Read the model definition and answer for the solid it produces. Units are mm, in the model's axes. Face numbers are marked on the shaded views. A direction names the side the tool comes from. Coordinates: 2 decimals unless noted, no trailing zeros. Write each loop counter-clockwise with the first axis right and the second up, starting at its lowest first coordinate (ties: lowest second). Pieces come first, ordered by that corner, then holes. Notation, with made-up numbers: (-37, -9.75) -> (-4, -9.75) arc R28 cw to (-4, 11.25) -> close; hole circle Ø9 at (22, -38.75). An arc over 180 degrees is marked (long way). One line per item, written item: value. Start each with the question number.
1. For the marked faces 4, 5 and 6, determine the directions among +Z, -Z, +X, -X, +Y, -Y from which every point of the face is accessible in a straight line to the end or side of a thin tool.
2. Find section C-C, the plane z = 4.25. Write down the section's boundary in (x, y).
3. Given P1, Ø1, axis at x = -5.5, z = 4.5, coming from the +Y side; P2, Ø2, axis at y = 6.5, z = 3, coming from the +X side, each flat-ended and moving along its own axis, determine where each tip first touches the part or whether it passes through.
4. Consider line 1 along Y through (x, z) = (5.25, 3.25); line 2 along Y through (x, z) = (-5, 0.5); line 3 along Z through (x, y) = (-0.75, -1.75). Determine where each line is inside the solid, lowest interval first.
5. For a pull along Y with two mould halves and no side action, classify the marked faces 1, 2 and 3 as pulls with the +Y half, pulls with the -Y half, needs draft (parallel to the pull), parting line crosses it, or undercut.
6. Find section B-B, the plane x = -1. Write down the section's boundary in (y, z).
7. Find section D-D, the plane y = 7. Write down the section's boundary in (x, z), and give its area (3 significant figures).
8. Find section A-A, the plane z = 5.3. Write down the section's boundary in (x, y), and give its area (3 significant figures).
```python
from build123d import *

# Parameters (mm, degrees)
F1_DEPTH      = 3
F2_DEPTH      = 6
F4_DEPTH      = 1.5
F4_DEPTH_BACK = 1.5


with BuildPart() as f1:
    # F0 (on Top) → F1 (new body)
    with BuildSketch(Plane.XY):
        with BuildLine():
            ThreePointArc((5.811145618, 2), (5.4091097712, 4.5797958998), (7.6000000059, 6))
            Line((7.6000000059, 6), (-7.5999999941, 6))
            ThreePointArc((-7.5999999941, 6), (-5.9029437231, 5.2970562728), (-5.2, 3.6))
            ThreePointArc((-5.2, 3.6), (-5.3579863385, 2.7436269845), (-5.811145618, 2))
            Line((-5.811145618, 2), (5.811145618, 2))
        make_face()
        with BuildLine():
            ThreePointArc((7.6, -6), (8.9856406461, -5.5595917942), (9.8627416998, -4.4))
            ThreePointArc((9.8627416998, -4.4), (8.9856406461, -3.2404082058), (7.6, -2.8))
            ThreePointArc((7.6, -2.8), (6.2143593539, -3.2404082058), (5.3372583002, -4.4))
            ThreePointArc((5.3372583002, -4.4), (6.2143593539, -5.5595917942), (7.6, -6))
        make_face()
        with BuildLine():
            ThreePointArc((9.8627416998, -4.4), (9.9654365432, -4.0058447489), (10, -3.6))
            ThreePointArc((10, -3.6), (8.0058447489, -1.2345634568), (5.3372583002, -2.8))
            Line((5.3372583002, -2.8), (7.6, -2.8))
            ThreePointArc((7.6, -2.8), (8.9856406461, -3.2404082058), (9.8627416998, -4.4))
        make_face()
        with BuildLine():
            ThreePointArc((7.6, -6), (6.2143593539, -5.5595917942), (5.3372583002, -4.4))
            ThreePointArc((5.3372583002, -4.4), (5.2, -5.2), (5.3372583002, -6))
            Line((5.3372583002, -6), (7.6, -6))
        make_face()
        with BuildLine():
            ThreePointArc((-5.3372583002, -4.4), (-6.2143593453, -5.5595917881), (-7.5999999788, -6))
            Line((-7.5999999788, -6), (-5.3372583002, -6))
            ThreePointArc((-5.3372583002, -6), (-5.2345634568, -5.6058447489), (-5.2, -5.2))
            ThreePointArc((-5.2, -5.2), (-5.2345634568, -4.7941552511), (-5.3372583002, -4.4))
        make_face()
        with BuildLine():
            ThreePointArc((-7.6, -2.8), (-8.9856406461, -3.2404082058), (-9.8627416998, -4.4))
            ThreePointArc((-9.8627416998, -4.4), (-8.9856406374, -5.5595918003), (-7.5999999788, -6))
            ThreePointArc((-7.5999999788, -6), (-6.2143593453, -5.5595917881), (-5.3372583002, -4.4))
            ThreePointArc((-5.3372583002, -4.4), (-6.2143593539, -3.2404082058), (-7.6, -2.8))
        make_face()
        with BuildLine():
            ThreePointArc((-5.3372583002, -2.8), (-8.0058447489, -1.2345634568), (-10, -3.6))
            ThreePointArc((-10, -3.6), (-9.9654365432, -4.0058447489), (-9.8627416998, -4.4))
            ThreePointArc((-9.8627416998, -4.4), (-8.9856406461, -3.2404082058), (-7.6, -2.8))
            Line((-7.6, -2.8), (-5.3372583002, -2.8))
        make_face()
        with BuildLine():
            ThreePointArc((-5.2, 3.6), (-5.9029437231, 5.2970562728), (-7.5999999941, 6))
            ThreePointArc((-7.5999999941, 6), (-9.2970562728, 5.2970562769), (-10, 3.6))
            ThreePointArc((-10, 3.6), (-9.8420136615, 2.7436269845), (-9.388854382, 2))
            Line((-9.388854382, 2), (-5.811145618, 2))
            ThreePointArc((-5.811145618, 2), (-5.3579863385, 2.7436269845), (-5.2, 3.6))
        make_face()
        with BuildLine():
            ThreePointArc((10, 3.6), (9.2970562769, 5.2970562728), (7.6000000059, 6))
            ThreePointArc((7.6000000059, 6), (5.4091097712, 4.5797958998), (5.811145618, 2))
            Line((5.811145618, 2), (9.388854382, 2))
            ThreePointArc((9.388854382, 2), (9.8420136615, 2.7436269845), (10, 3.6))
        make_face()
        with BuildLine():
            ThreePointArc((5.3372583002, -4.4), (5.2, -3.6), (5.3372583002, -2.8))
            Line((5.3372583002, -2.8), (-5.3372583002, -2.8))
            ThreePointArc((-5.3372583002, -2.8), (-5.2345634568, -3.1941552511), (-5.2, -3.6))
            ThreePointArc((-5.2, -3.6), (-5.2345634568, -4.0058447489), (-5.3372583002, -4.4))
            ThreePointArc((-5.3372583002, -4.4), (-5.2345634568, -4.7941552511), (-5.2, -5.2))
            ThreePointArc((-5.2, -5.2), (-5.2345634568, -5.6058447489), (-5.3372583002, -6))
            Line((-5.3372583002, -6), (5.3372583002, -6))
            ThreePointArc((5.3372583002, -6), (5.2, -5.2), (5.3372583002, -4.4))
        make_face()
        with BuildLine():
            ThreePointArc((-5.2, -3.6), (-5.2345634568, -3.1941552511), (-5.3372583002, -2.8))
            Line((-5.3372583002, -2.8), (-7.6, -2.8))
            ThreePointArc((-7.6, -2.8), (-6.2143593539, -3.2404082058), (-5.3372583002, -4.4))
            ThreePointArc((-5.3372583002, -4.4), (-5.2345634568, -4.0058447489), (-5.2, -3.6))
        make_face()
        with BuildLine():
            Line((7.6, -2.8), (5.3372583002, -2.8))
            ThreePointArc((5.3372583002, -2.8), (5.2, -3.6), (5.3372583002, -4.4))
            ThreePointArc((5.3372583002, -4.4), (6.2143593539, -3.2404082058), (7.6, -2.8))
        make_face()
        with BuildLine():
            ThreePointArc((9.388854382, 2), (7.6, 1.2), (5.811145618, 2))
            Line((5.811145618, 2), (-5.811145618, 2))
            ThreePointArc((-5.811145618, 2), (-7.6, 1.2), (-9.388854382, 2))
            Line((-9.388854382, 2), (-10, 2))
            Line((-10, 2), (-10, -3.6))
            ThreePointArc((-10, -3.6), (-8.0058447489, -1.2345634568), (-5.3372583002, -2.8))
            Line((-5.3372583002, -2.8), (5.3372583002, -2.8))
            ThreePointArc((5.3372583002, -2.8), (8.0058447489, -1.2345634568), (10, -3.6))
            Line((10, -3.6), (10, 2))
            Line((10, 2), (9.388854382, 2))
        make_face()
        with BuildLine():
            Line((9.388854382, 2), (5.811145618, 2))
            ThreePointArc((5.811145618, 2), (7.6, 1.2), (9.388854382, 2))
        make_face()
        with BuildLine():
            ThreePointArc((-9.388854382, 2), (-7.6, 1.2), (-5.811145618, 2))
            Line((-5.811145618, 2), (-9.388854382, 2))
        make_face()
        with BuildLine():
            ThreePointArc((-9.388854382, 2), (-9.8420136615, 2.7436269845), (-10, 3.6))
            Line((-10, 3.6), (-10, 2))
            Line((-10, 2), (-9.388854382, 2))
        make_face()
        with BuildLine():
            Line((10, 2), (10, 3.6))
            ThreePointArc((10, 3.6), (9.8420136615, 2.7436269845), (9.388854382, 2))
            Line((9.388854382, 2), (10, 2))
        make_face()
    extrude(amount=F1_DEPTH)

    # F0 (on Top) → F2 (join)
    with BuildSketch(Plane.XY):
        with BuildLine():
            ThreePointArc((5.3372583002, -4.4), (5.2, -3.6), (5.3372583002, -2.8))
            Line((5.3372583002, -2.8), (-5.3372583002, -2.8))
            ThreePointArc((-5.3372583002, -2.8), (-5.2345634568, -3.1941552511), (-5.2, -3.6))
            ThreePointArc((-5.2, -3.6), (-5.2345634568, -4.0058447489), (-5.3372583002, -4.4))
            ThreePointArc((-5.3372583002, -4.4), (-5.2345634568, -4.7941552511), (-5.2, -5.2))
            ThreePointArc((-5.2, -5.2), (-5.2345634568, -5.6058447489), (-5.3372583002, -6))
            Line((-5.3372583002, -6), (5.3372583002, -6))
            ThreePointArc((5.3372583002, -6), (5.2, -5.2), (5.3372583002, -4.4))
        make_face()
        with BuildLine():
            ThreePointArc((-7.6, -2.8), (-8.9856406461, -3.2404082058), (-9.8627416998, -4.4))
            ThreePointArc((-9.8627416998, -4.4), (-8.9856406374, -5.5595918003), (-7.5999999788, -6))
            ThreePointArc((-7.5999999788, -6), (-6.2143593453, -5.5595917881), (-5.3372583002, -4.4))
            ThreePointArc((-5.3372583002, -4.4), (-6.2143593539, -3.2404082058), (-7.6, -2.8))
        make_face()
        with BuildLine():
            ThreePointArc((-5.3372583002, -4.4), (-6.2143593453, -5.5595917881), (-7.5999999788, -6))
            Line((-7.5999999788, -6), (-5.3372583002, -6))
            ThreePointArc((-5.3372583002, -6), (-5.2345634568, -5.6058447489), (-5.2, -5.2))
            ThreePointArc((-5.2, -5.2), (-5.2345634568, -4.7941552511), (-5.3372583002, -4.4))
        make_face()
        with BuildLine():
            ThreePointArc((-5.2, -3.6), (-5.2345634568, -3.1941552511), (-5.3372583002, -2.8))
            Line((-5.3372583002, -2.8), (-7.6, -2.8))
            ThreePointArc((-7.6, -2.8), (-6.2143593539, -3.2404082058), (-5.3372583002, -4.4))
            ThreePointArc((-5.3372583002, -4.4), (-5.2345634568, -4.0058447489), (-5.2, -3.6))
        make_face()
        with BuildLine():
            ThreePointArc((7.6, -6), (8.9856406461, -5.5595917942), (9.8627416998, -4.4))
            ThreePointArc((9.8627416998, -4.4), (8.9856406461, -3.2404082058), (7.6, -2.8))
            ThreePointArc((7.6, -2.8), (6.2143593539, -3.2404082058), (5.3372583002, -4.4))
            ThreePointArc((5.3372583002, -4.4), (6.2143593539, -5.5595917942), (7.6, -6))
        make_face()
        with BuildLine():
            ThreePointArc((7.6, -6), (6.2143593539, -5.5595917942), (5.3372583002, -4.4))
            ThreePointArc((5.3372583002, -4.4), (5.2, -5.2), (5.3372583002, -6))
            Line((5.3372583002, -6), (7.6, -6))
        make_face()
        with BuildLine():
            Line((7.6, -2.8), (5.3372583002, -2.8))
            ThreePointArc((5.3372583002, -2.8), (5.2, -3.6), (5.3372583002, -4.4))
            ThreePointArc((5.3372583002, -4.4), (6.2143593539, -3.2404082058), (7.6, -2.8))
        make_face()
        with BuildLine():
            ThreePointArc((-5.2, 3.6), (-5.9029437231, 5.2970562728), (-7.5999999941, 6))
            ThreePointArc((-7.5999999941, 6), (-9.2970562728, 5.2970562769), (-10, 3.6))
            ThreePointArc((-10, 3.6), (-9.8420136615, 2.7436269845), (-9.388854382, 2))
            Line((-9.388854382, 2), (-5.811145618, 2))
            ThreePointArc((-5.811145618, 2), (-5.3579863385, 2.7436269845), (-5.2, 3.6))
        make_face()
        with BuildLine():
            ThreePointArc((5.811145618, 2), (5.4091097712, 4.5797958998), (7.6000000059, 6))
            Line((7.6000000059, 6), (-7.5999999941, 6))
            ThreePointArc((-7.5999999941, 6), (-5.9029437231, 5.2970562728), (-5.2, 3.6))
            ThreePointArc((-5.2, 3.6), (-5.3579863385, 2.7436269845), (-5.811145618, 2))
            Line((-5.811145618, 2), (5.811145618, 2))
        make_face()
        with BuildLine():
            ThreePointArc((10, 3.6), (9.2970562769, 5.2970562728), (7.6000000059, 6))
            ThreePointArc((7.6000000059, 6), (5.4091097712, 4.5797958998), (5.811145618, 2))
            Line((5.811145618, 2), (9.388854382, 2))
            ThreePointArc((9.388854382, 2), (9.8420136615, 2.7436269845), (10, 3.6))
        make_face()
        with BuildLine():
            Line((10, 2), (10, 3.6))
            ThreePointArc((10, 3.6), (9.8420136615, 2.7436269845), (9.388854382, 2))
            Line((9.388854382, 2), (10, 2))
        make_face()
        with BuildLine():
            ThreePointArc((-9.388854382, 2), (-9.8420136615, 2.7436269845), (-10, 3.6))
            Line((-10, 3.6), (-10, 2))
            Line((-10, 2), (-9.388854382, 2))
        make_face()
    extrude(amount=F2_DEPTH)

    # F3 (on Right) → F4 (join, two sides)
    with BuildSketch(Plane.YZ) as f4_sk:
        Polygon((6, 1), (6, 0), (12, 0), (12, 6), (6, 6), (6, 5), (11, 5), (11, 1), align=None)
    extrude(amount=F4_DEPTH)
    extrude(f4_sk.sketch, amount=-F4_DEPTH_BACK)


solid = f1.part
```
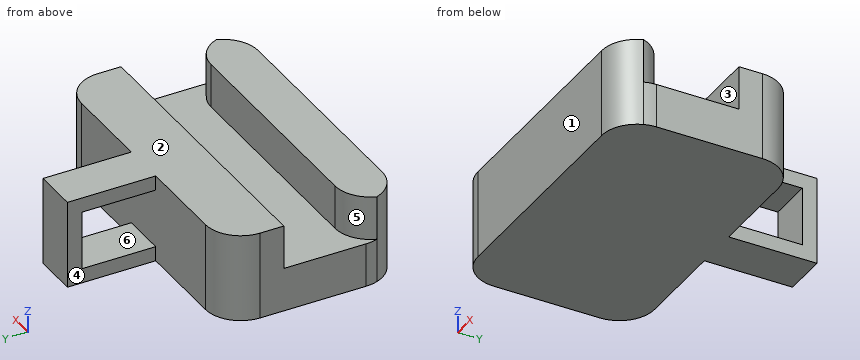
Answer block:
1. face 4: +Z, -Z, -X, +Y
1. face 5: +Z, -X
1. face 6: +X, -X
2. outline: (-10, 2) -> (10, 2) -> (10, 3.6) arc R2.4 ccw to (7.6, 6) -> (-7.6, 6) arc R2.4 ccw to (-10, 3.6) -> close; (-9.86, -4.4) arc R2.4 ccw to (-7.6, -6) -> (7.6, -6) arc R2.4 ccw to (9.86, -4.4) arc R2.4 ccw to (7.6, -2.8) -> (-7.6, -2.8) arc R2.4 ccw to start; (-1.5, 11) -> (1.5, 11) -> (1.5, 12) -> (-1.5, 12) -> close
3. P1: stops at y = 6
3. P2: stops at x = 9.07
4. line 1: y = -6 to -2.8, 2 to 6
4. line 2: y = -6 to 6
4. line 3: z = 0 to 3
5. face 1: pulls with the -Y half
5. face 2: needs draft
5. face 3: undercut
6. outline: (-6, 0) -> (12, 0) -> (12, 6) -> (2, 6) -> (2, 3) -> (-2.8, 3) -> (-2.8, 6) -> (-6, 6) -> close; hole (6, 1) -> (11, 1) -> (11, 5) -> (6, 5) -> close
7. outline: (-1.5, 0) -> (1.5, 0) -> (1.5, 1) -> (-1.5, 1) -> close; (-1.5, 5) -> (1.5, 5) -> (1.5, 6) -> (-1.5, 6) -> close
7. area: 6.00 mm2
8. outline: (-10, 2) -> (10, 2) -> (10, 3.6) arc R2.4 ccw to (7.6, 6) -> (1.5, 6) -> (1.5, 12) -> (-1.5, 12) -> (-1.5, 6) -> (-7.6, 6) arc R2.4 ccw to (-10, 3.6) -> close; (-9.86, -4.4) arc R2.4 ccw to (-7.6, -6) -> (7.6, -6) arc R2.4 ccw to (9.86, -4.4) arc R2.4 ccw to (7.6, -2.8) -> (-7.6, -2.8) arc R2.4 ccw to start
8. area: 155 mm2
